Source: CAD feature listing. Evaluate the final solid. Frame: model axes, mm. Face numbers are marked on the shaded views. A direction names the side the tool comes from. Give positions to 0.01 mm unless a question says otherwise; leave off trailing zeros. Order: outer loops, then holes, each group sorted by start corner. A loop starts at its lowest first (then second) coordinate and runs counter-clockwise, first axis right, second up.
1) Draft query along Y for the marked faces 1, 2, 3 and 4. Return one class per face: released by +Y, released by -Y, zero draft, split by the parting line, or undercut.
2) Section D-D, the plane x = 2. Give the number of separate pieces and of enclosed holes in the cut face, plus the area to 3 significant figures.
3) Material intervals for line 1 (Y direction, x = 8.5, z = 27.5); line 2 (Z direction, x = 0, y = -52); line 3 (Z direction, x = 0, y = -19.25), sorted ascending.
4) Section C-C, the plane y = -3. Return loops of the section in (x, z), plus the area to 3 significant figures.
5) Section B-B, the plane z = 79. Return loops of the section in (x, y).
6) Access query for the marked faces 5 and 6. Directions: +Z, -Z, +X, -X, +Y, -Y. A direction counts if a zero-diameter tool reaches every point of the face in a straight line with its end or side. Return the directions, or none.
7) Section A-A, the plane z = -6.5. Return loops of the section in (x, y).
8) First-contact query: P1, Ø2, axis at x = -17, y = 29.5, coming from the +Z side; P2, Ø3, axis at x = 19.5, z = -38, coming from the -Y side; P3, Ø5, axis at y = 26.5, z = -10, coming from the +X side. Flat tips, straight axial feed; report the tip coordinate or a pass-through.
```python
from build123d import *

# Parameters (mm, degrees)
F1_DEPTH = 90
F2_DEPTH = 75
F4_DEPTH = 90
F6_W     = 41
F6_H     = 21
F7_DEPTH = 71
F8_R     = 10.5
F9_DEPTH = 200


# Not quite as in the source:
# - a feature names something its author has since deleted; it is built from what else it names


with BuildPart() as f1:
    # F0 (on Top) → F1 (new body)
    with BuildSketch(Plane.XY):
        with BuildLine():
            ThreePointArc((30, -51.9615242271), (51.9615242271, -30), (60, 0))
            ThreePointArc((60, 0), (51.9615242271, 30), (30, 51.9615242271))
            ThreePointArc((30, 51.9615242271), (15.5291427062, 57.9555495773), (0, 60))
            ThreePointArc((0, 60), (-15.5291427062, 57.9555495773), (-30, 51.9615242271))
            ThreePointArc((-30, 51.9615242271), (-60, 0), (-30, -51.9615242271))
            ThreePointArc((-30, -51.9615242271), (-15.5291427062, -57.9555495773), (0, -60))
            ThreePointArc((0, -60), (15.5291427062, -57.9555495773), (30, -51.9615242271))
        make_face()
        with BuildLine():
            ThreePointArc((-8, 22.627416998), (0, 24), (8, 22.627416998))
            Line((8, 22.627416998), (8, 13))
            ThreePointArc((8, 13), (9.4644660941, 9.4644660941), (13, 8))
            Line((13, 8), (22.627416998, 8))
            ThreePointArc((22.627416998, 8), (24, 0), (22.627416998, -8))
            Line((22.627416998, -8), (13, -8))
            ThreePointArc((13, -8), (9.4644660941, -9.4644660941), (8, -13))
            Line((8, -13), (8, -22.627416998))
            ThreePointArc((8, -22.627416998), (0, -24), (-8, -22.627416998))
            Line((-8, -22.627416998), (-8, -13))
            ThreePointArc((-8, -13), (-9.4644660941, -9.4644660941), (-13, -8))
            Line((-13, -8), (-22.627416998, -8))
            ThreePointArc((-22.627416998, -8), (-24, 0), (-22.627416998, 8))
            Line((-22.627416998, 8), (-13, 8))
            ThreePointArc((-13, 8), (-9.4644660941, 9.4644660941), (-8, 13))
            Line((-8, 13), (-8, 22.627416998))
        make_face(mode=Mode.SUBTRACT)
        with BuildLine():
            ThreePointArc((0, 60), (15.5291427062, 57.9555495773), (30, 51.9615242271))
            Line((30, 51.9615242271), (30, 60))
            Line((30, 60), (0, 60))
        make_face()
        with BuildLine():
            Line((30, -60), (30, -51.9615242271))
            ThreePointArc((30, -51.9615242271), (15.5291427062, -57.9555495773), (0, -60))
            Line((0, -60), (30, -60))
        make_face()
        with BuildLine():
            ThreePointArc((-30, 51.9615242271), (-15.5291427062, 57.9555495773), (0, 60))
            Line((0, 60), (-30, 60))
            Line((-30, 60), (-30, 51.9615242271))
        make_face()
        with BuildLine():
            Line((-30, -60), (0, -60))
            ThreePointArc((0, -60), (-15.5291427062, -57.9555495773), (-30, -51.9615242271))
            Line((-30, -51.9615242271), (-30, -60))
        make_face()
        with BuildLine():
            Line((8, 13), (8, 22.627416998))
            ThreePointArc((8, 22.627416998), (0, 24), (-8, 22.627416998))
            Line((-8, 22.627416998), (-8, 13))
            ThreePointArc((-8, 13), (-9.4644660941, 9.4644660941), (-13, 8))
            Line((-13, 8), (-22.627416998, 8))
            ThreePointArc((-22.627416998, 8), (-24, 0), (-22.627416998, -8))
            Line((-22.627416998, -8), (-13, -8))
            ThreePointArc((-13, -8), (-9.4644660941, -9.4644660941), (-8, -13))
            Line((-8, -13), (-8, -22.627416998))
            ThreePointArc((-8, -22.627416998), (0, -24), (8, -22.627416998))
            Line((8, -22.627416998), (8, -13))
            ThreePointArc((8, -13), (9.4644660941, -9.4644660941), (13, -8))
            Line((13, -8), (22.627416998, -8))
            ThreePointArc((22.627416998, -8), (24, 0), (22.627416998, 8))
            Line((22.627416998, 8), (13, 8))
            ThreePointArc((13, 8), (9.4644660941, 9.4644660941), (8, 13))
        make_face()
    extrude(amount=F1_DEPTH)

    # F0 (on Top) → F2 (join)
    with BuildSketch(Plane.XY):
        with BuildLine():
            ThreePointArc((30, -51.9615242271), (51.9615242271, -30), (60, 0))
            ThreePointArc((60, 0), (51.9615242271, 30), (30, 51.9615242271))
            ThreePointArc((30, 51.9615242271), (15.5291427062, 57.9555495773), (0, 60))
            ThreePointArc((0, 60), (-15.5291427062, 57.9555495773), (-30, 51.9615242271))
            ThreePointArc((-30, 51.9615242271), (-60, 0), (-30, -51.9615242271))
            ThreePointArc((-30, -51.9615242271), (-15.5291427062, -57.9555495773), (0, -60))
            ThreePointArc((0, -60), (15.5291427062, -57.9555495773), (30, -51.9615242271))
        make_face()
        with BuildLine():
            ThreePointArc((-8, 22.627416998), (0, 24), (8, 22.627416998))
            Line((8, 22.627416998), (8, 13))
            ThreePointArc((8, 13), (9.4644660941, 9.4644660941), (13, 8))
            Line((13, 8), (22.627416998, 8))
            ThreePointArc((22.627416998, 8), (24, 0), (22.627416998, -8))
            Line((22.627416998, -8), (13, -8))
            ThreePointArc((13, -8), (9.4644660941, -9.4644660941), (8, -13))
            Line((8, -13), (8, -22.627416998))
            ThreePointArc((8, -22.627416998), (0, -24), (-8, -22.627416998))
            Line((-8, -22.627416998), (-8, -13))
            ThreePointArc((-8, -13), (-9.4644660941, -9.4644660941), (-13, -8))
            Line((-13, -8), (-22.627416998, -8))
            ThreePointArc((-22.627416998, -8), (-24, 0), (-22.627416998, 8))
            Line((-22.627416998, 8), (-13, 8))
            ThreePointArc((-13, 8), (-9.4644660941, 9.4644660941), (-8, 13))
            Line((-8, 13), (-8, 22.627416998))
        make_face(mode=Mode.SUBTRACT)
    extrude(amount=-F2_DEPTH)

    # F3 (on face) → F4 (cut)
    with BuildSketch(Plane.XY.offset(90)):
        with BuildLine():
            ThreePointArc((20.2484567313, -15.5), (24.1514559256, -8.1827365029), (25.5, 0))
            ThreePointArc((25.5, 0), (24.1514559256, 8.1827365029), (20.2484567313, 15.5))
            Line((20.2484567313, 15.5), (-20.2484567313, 15.5))
            ThreePointArc((-20.2484567313, 15.5), (-25.5, 0), (-20.2484567313, -15.5))
            Line((-20.2484567313, -15.5), (20.2484567313, -15.5))
        make_face()
    extrude(amount=-F4_DEPTH, mode=Mode.SUBTRACT)

    # F6 (on face) → F7 (cut)
    with BuildSketch(Plane.XY.offset(90)):
        with Locations((0, 37.75)):
            Rectangle(F6_W, F6_H)
        with Locations((0, -37.75)):
            Rectangle(F6_W, F6_H)
    extrude(amount=-F7_DEPTH, mode=Mode.SUBTRACT)

    # F8 (on face) → F9 (cut)
    with BuildSketch(Plane(origin=(0, 60, 0), x_dir=(-1, 0, 0), z_dir=(0, 1, 0))):
        with Locations((0, 41)):
            Circle(F8_R)
    extrude(amount=-F9_DEPTH, mode=Mode.SUBTRACT)


solid = f1.part
```
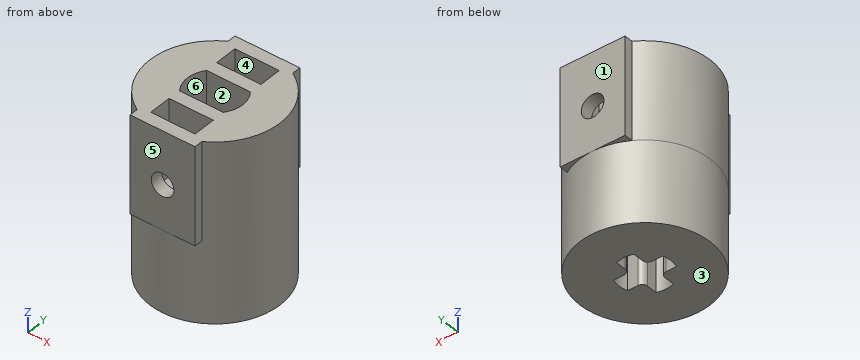
From the geometry:
1. face 1: released by +Y
1. face 2: undercut
1. face 3: zero draft
1. face 4: undercut
2. separate pieces: 6
2. enclosed holes: 0
2. area: 9,470 mm2
3. line 1: y = -60 to -48.25, -27.25 to -15.5, 15.5 to 27.25, 48.25 to 60
3. line 2: z = -75 to 30.5, 51.5 to 90
3. line 3: z = 0 to 30.5, 51.5 to 90
4. outline: (-59.92, -75) - (-23.81, -75) - (-23.81, 0) - (-25.32, 0) - (-25.32, 90) - (-59.92, 90) - close; (23.81, -75) - (59.92, -75) - (59.92, 90) - (25.32, 90) - (25.32, 0) - (23.81, 0) - close
4. area: 11,600 mm2
5. outline: (-30, -60) - (30, -60) - (30, -51.96) arc R60 ccw to (30, 51.96) - (30, 60) - (-30, 60) - (-30, 51.96) arc R60 ccw to (-30, -51.96) - close; hole (-20.5, -48.25) - (20.5, -48.25) - (20.5, -27.25) - (-20.5, -27.25) - close; hole (-20.5, 27.25) - (20.5, 27.25) - (20.5, 48.25) - (-20.5, 48.25) - close; hole (-20.25, -15.5) - (20.25, -15.5) arc R25.5 ccw to (20.25, 15.5) - (-20.25, 15.5) arc R25.5 ccw to start
6. face 5: +Z, -Z, +X, -X, -Y
6. face 6: +Z
7. outline: circle Ø120 at (0, 0); hole (-22.63, -8) - (-13, -8) arc R5 cw to (-8, -13) - (-8, -22.63) arc R24 ccw to (8, -22.63) - (8, -13) arc R5 cw to (13, -8) - (22.63, -8) arc R24 ccw to (22.63, 8) - (13, 8) arc R5 cw to (8, 13) - (8, 22.63) arc R24 ccw to (-8, 22.63) - (-8, 13) arc R5 cw to (-13, 8) - (-22.63, 8) arc R24 ccw to start
8. P1: stops at z = 19
8. P2: stops at y = -57.24
8. P3: stops at x = 54.99
